from build123d import *

# Parameters (mm, degrees)
SKETCH_1_W          = 40
SKETCH_1_H          = 14
EXTRUDE_1_DEPTH     = 60
SKETCH_6_W          = 36
SKETCH_6_H          = 10
CUT_EXTRUDE_2_DEPTH = 55
SKETCH_7_W          = 40
SKETCH_7_H          = 10
CUT_EXTRUDE_3_DEPTH = 7


with BuildPart() as part:
    # 草图1 → 凸台-拉伸1 (new body)
    with BuildSketch(Plane(origin=(0, 0, 0), x_dir=(1, 0, 0), z_dir=(0, 1, 0))):
        with Locations((20, 7)):
            Rectangle(SKETCH_1_W, SKETCH_1_H)
    extrude(amount=EXTRUDE_1_DEPTH)

    # 草图6 → 切除-拉伸2 (cut)
    with BuildSketch(Plane(origin=(0, 60, 0), x_dir=(1, 0, 0), z_dir=(0, 1, 0))):
        with Locations((20, 7)):
            Rectangle(SKETCH_6_W, SKETCH_6_H)
    extrude(amount=-CUT_EXTRUDE_2_DEPTH, mode=Mode.SUBTRACT)

    # 草图7 → 切除-拉伸3 (cut)
    with BuildSketch(Plane.XY):
        with Locations((20, 55)):
            Rectangle(SKETCH_7_W, SKETCH_7_H)
    extrude(amount=-CUT_EXTRUDE_3_DEPTH, mode=Mode.SUBTRACT)


solid = part.part
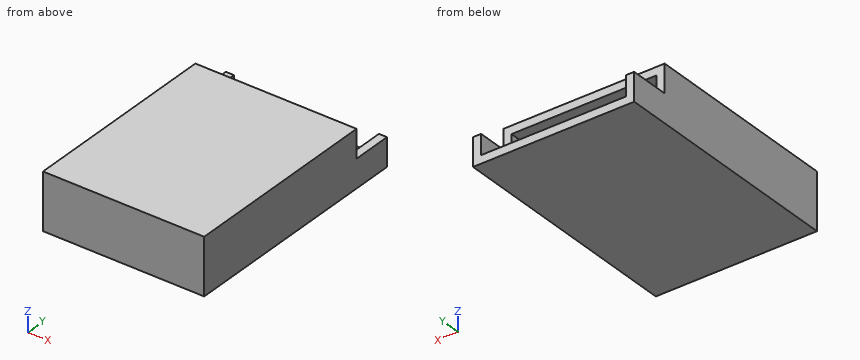
Could you check a few things on this model? Use its own coordinates, in mm. Coordinates: 2 decimals unless noted, no trailing zeros. Loops run counter-clockwise (first coordinate to the right, second up) from the corner with the lowest first, then second, coordinate; pieces in that order, holes last.
1. Imagine slicing it at A-A (x = 11.5). Please give me the cut outline in (y, z).
2. Imagine slicing it at B-B (y = 23). Please give me the cut outline in (x, z), and give its area (3 significant figures).
3. For P1, Ø8, axis at y = 41.5, z = -5, coming from the -X side; P2, Ø0.6, axis at x = 39.5, y = 56, coming from the +Z side; P3, Ø2, axis at x = 6.5, z = -8, coming from the +Y side; P4, Ø7.5, axis at x = 21, z = -3, coming from the +Y side, each with a flat end and sliding along its axis, tell me the tip position at first contact or that it passes through.
4. I need wall thicknesses on L1, parallel to X at y = 41, z = -7; L2, parallel to Z at x = 8.5, y = 27.5; L3, parallel to Z at x = 30, y = 57. Which ranges of each line are inside material? Lowest first, please.
5. Imagine slicing it at C-C (z = -10). Please give me the cut outline in (x, y), and give its area (3 significant figures).
Computed values:
1. outline: (0, -14) - (60, -14) - (60, -12) - (5, -12) - (5, -2) - (50, -2) - (50, 0) - (0, 0) - close
2. outline: (0, -14) - (40, -14) - (40, 0) - (0, 0) - close; hole (2, -12) - (38, -12) - (38, -2) - (2, -2) - close
2. area: 200 mm2
3. P1: stops at x = 0
3. P2: stops at z = -7
3. P3: stops at y = 5
3. P4: stops at y = 50
4. L1: x = 0 to 2, 38 to 40
4. L2: z = -14 to -12, -2 to 0
4. L3: z = -14 to -12
5. outline: (0, 0) - (40, 0) - (40, 60) - (38, 60) - (38, 5) - (2, 5) - (2, 60) - (0, 60) - close
5. area: 420 mm2
